```python
from build123d import *

# Parameters (mm, degrees)
SKETCH1_R               = 141
BOSS_EXTRUDE1_DEPTH     = 3.5
SKETCH2_R               = 141
SKETCH2_R_2             = 131
BOSS_EXTRUDE2_DEPTH     = 8
SKETCH5_R               = 2
CUT_EXTRUDE3_DEPTH      = 5
CUT_EXTRUDE3_DEPTH_BACK = 15


with BuildPart() as part:
    # Sketch1 → Boss-Extrude1 (new body)
    with BuildSketch(Plane(origin=(0, 0, 0), x_dir=(1, 0, 0), z_dir=(0, 1, 0))):
        with Locations(Location((0, 0, 0), (0, 0, 270))):
            Circle(SKETCH1_R)
    extrude(amount=BOSS_EXTRUDE1_DEPTH)

    # Sketch2 → Boss-Extrude2 (add)
    with BuildSketch(Plane(origin=(0, 3.5, 0), x_dir=(1, 0, 0), z_dir=(0, 1, 0))):
        with Locations(Location((0, 0, 0), (0, 0, 270))):
            Circle(SKETCH2_R)
        with Locations(Location((0, 0, 0), (0, 0, 270))):
            Circle(SKETCH2_R_2, mode=Mode.SUBTRACT)
    extrude(amount=BOSS_EXTRUDE2_DEPTH)

    # Cut-Sweep1: sweep along a path in Sketch3
    with BuildLine(Plane(origin=(0, 11.5, 0), x_dir=(1, 0, 0), z_dir=(0, 1, 0))) as cut_sweep1_path:
        CenterArc((0, 0), 136, 0, 360)
    # Sketch5 → Cut-Sweep1 (sweep, cut)
    with BuildSketch(Plane(origin=(0, 0, 0), x_dir=(0.9955256364380607, 0, -0.09449183665584275), z_dir=(0.09449183665584275, 0, 0.9955256364380607))):
        with Locations((136, 10.2)):
            Circle(SKETCH5_R)
    sweep(path=cut_sweep1_path.line, mode=Mode.SUBTRACT)

    # Sketch6 → Cut-Extrude3 (cut, two sides: drawn at the far end of the back side and taken through both)
    with BuildSketch(Plane(origin=(130.413858373, 0, -12.378430602), x_dir=(0.09449183665584276, 0, 0.9955256364380607), z_dir=(-0.9955256364380607, 0, 0.09449183665584276)).offset(-CUT_EXTRUDE3_DEPTH_BACK)):
        with BuildLine():
            Line((1, 3.599112528), (-1, 3.599112528))
            ThreePointArc((-1, 3.599112528), (-2.8, 5.399112528), (-1, 7.199112528))
            Line((-1, 7.199112528), (1, 7.199112528))
            ThreePointArc((1, 7.199112528), (2.8, 5.399112528), (1, 3.599112528))
        make_face()
    extrude(amount=CUT_EXTRUDE3_DEPTH + CUT_EXTRUDE3_DEPTH_BACK, mode=Mode.SUBTRACT)


solid = part.part
```
Build history of the part. All positions in model axes, mm. A direction names the side the tool comes from. Coordinates: 2 decimals unless noted, no trailing zeros. Order: outer loops, then holes, each group sorted by start corner. A loop starts at its lowest first (then second) coordinate and runs counter-clockwise, first axis right, second up. Notation, with made-up numbers: M 46.5,79 L 54.5,79 A17 cw 54.5,83 Z; hole C 15.5,70.5 d11. An arc over 180 degrees is marked long. One line per question, with ' | ' between items. Start each with the question number.
1. Flat gauge pins, fed straight in: P1, Ø5, axis at x = -4, z = 53.5, coming from the +Y side; P2, Ø0.9, axis at x = 136, z = -12.5, coming from the +Y side; P3, Ø5, axis at x = 80.5, y = 8.5, coming from the +Z side. Where does each tip first touch, or does it go through?
2. Tool access for faces 4 (the face through (-129, 11.5, 29)), 5 (the face through (39.35, 7.44, 124.95)): list every direction of +Z, -Z, +X, -X, +Y, -Y with a clear straight run to the whole face (end or side of a thin tool).
3. Cut at B-B (x = 0). Write the cut outline in (y, z), plus the area to 3 significant figures.
4. Cut at A-A (z = 0). Write the cut outline in (x, y), plus the area to 3 significant figures.
5. Wall check: line 1 along X through (y, z) = (9, 0); line 2 along X through (y, z) = (10, 0); line 3 along Y through (x, z) = (111.5, -3). Give the ranges that are in metal, low to high. Write a range as [from, to].
6. Mould opens along X. For faces 1 (the face through (2, 3.5, -2)), 2 (the face through (-85.8, 5.67, -111.89)), 3 (the face through (2, 0, -2)) say: +X half, -X half, draft (parallel to the pull), parting line (faces both ways), or undercut.
The answers:
1) P1: stops at y = 3.5 | P2: stops at y = 8.48 | P3: stops at z = 117.46
2) face 4: +Z, -Z, +X, -X, +Y | face 5: +Y
3) outline: M 0,-141 L 11.5,-141 L 11.5,-137.52 A2 cw long 11.5,-134.48 L 11.5,-131 L 3.5,-131 L 3.5,131 L 11.5,131 L 11.5,134.48 A2 cw long 11.5,137.52 L 11.5,141 L 0,141 Z | area: 1,120 mm2
4) outline: M -141,0 L 141,0 L 141,11.5 L 137.52,11.5 A2 cw long 134.48,11.5 L 131,11.5 L 131,3.5 L -131,3.5 L -131,11.5 L -134.48,11.5 A2 cw long -137.52,11.5 L -141,11.5 Z | area: 1,120 mm2
5) line 1: x = [-141, -137.6], [-134.4, -131], [131, 134.4], [137.6, 141] | line 2: x = [-141, -137.99], [-134.01, -131], [131, 134.01], [137.99, 141] | line 3: y = [0, 3.5]
6) face 1: undercut | face 2: parting line | face 3: draft
